Autodesk Inventor part; units mm, degrees
ref_plane "YZ Plane" through (0, 0, 0) normal (1, 0, 0) x (0, 1, 0)
ref_plane "XZ Plane" through (0, 0, 0) normal (0, 1, 0) x (-1, 0, 0)
ref_plane "XY Plane" through (0, 0, 0) normal (0, 0, 1) x (1, 0, 0)
sketch "Sketch1" plane through (0, 0, 0) normal (1, 0, 0) x (0, 1, 0)
  line L0 (0, 0) -> (3.5, 0)
  arc A0 (6.3262, -0.7277) -> (3.5, 0) centre (3.7831, -4.7528) ccw
  arc A1 (6.3262, -0.7277) -> (9.2314, -2.0228) centre (10.456, 4.6303) ccw
  line L1 (0, 0) -> (0, 0.25)
  line L2 (0, 0.25) -> (3.5, 0.25)
  line L3 (6.3262, -0.7277) -> (6.3262, -0.4777)
  line L4 (9.2314, -2.0228) -> (9.2314, -1.7728)
  arc A2 (6.3262, -0.4777) -> (3.5, 0.25) centre (3.658, -4.9886) ccw
  arc A3 (6.3262, -0.4777) -> (9.2314, -1.7728) centre (10.4213, 4.8026) ccw
  dimension "d0" = 3.5
  dimension "d1" = 0.25
  dimension "d2" = 3.5
  dimension "d3" = 0.25
  dimension "d4" = 0.25
extrude "Extrusion1" add sketch "Sketch1" along normal blind 5
properties part number "ribbonCable"
Verification items for the finished model (mm, model axes). Coordinates: 2 decimals unless noted, no trailing zeros. Order: outer loops, then holes, each group sorted by start corner. A loop starts at its lowest first (then second) coordinate and runs counter-clockwise, first axis right, second up. Notation, with made-up numbers: (69, 27.5) -> (128, 27.5) arc R7 cw to (128, 32.5) -> close; hole circle Ø5 at (7.25, 10.5). An arc over 180 degrees is marked (long way). Use CSV: the item, a comma, the result in double quotes. Start each with the question number.
Q1. Section check B-B, the plane z = 0.15. Record the cut outline in (x, y), and give its area (3 significant figures).
Q2. Depth check by flat-ended pin: P1, Ø3, axis at x = 1.5, y = 2, coming from the -Z side; P2, Ø3, axis at x = 1, y = 4.5, coming from the -Z side; P3, Ø1, axis at x = 2.5, y = 2, coming from the +Z side. Enter the tip coordinate at first touch or a pass-through.
Q3. Thickness scan on line 1 along Z through (x, y) = (2.1, 3.5); line 2 along Y through (x, z) = (2.75, -0.4). Record the ranges inside material, lowest first.
Q4. Section check A-A, the plane x = 0.3. Record the cut outline in (y, z), and give its area (3 significant figures).
Q5. Draft check along Y on faces 1 (the cylindrical face through (2.465, 7.722, -1.558)), 2 (the cylindrical face through (2.5, 7.7, -1.3)), 3 (the flat face through (2, 2, 0)). Enter one of: +Y half, -Y half, draft (parallel to the pull), parting line (faces both ways), or undercut.
Q6. Section check C-C, the plane y = 7.75. Record the cut outline in (x, z).
Returned:
1,outline,"(0, 0) -> (5, 0) -> (5, 4.69) -> (0, 4.69) -> close"
1,area,"23.4 mm^2"
2,P1,"stops at z = 0"
2,P2,"stops at z = -0.54"
2,P3,"stops at z = 0.25"
3,line 1,"z = 0 to 0.25"
3,line 2,"y = 5.71 to 6.19"
4,outline,"(0, 0) -> (3.5, 0) arc R4.76 cw to (6.33, -0.73) arc R6.76 ccw to (9.23, -2.02) -> (9.23, -1.77) arc R6.68 cw to (6.33, -0.48) arc R5.24 ccw to (3.5, 0.25) -> (0, 0.25) -> close"
4,area,"2.26 mm^2"
5,face 1,"-Y half"
5,face 2,"+Y half"
5,face 3,"draft"
6,outline,"(0, -1.57) -> (5, -1.57) -> (5, -1.32) -> (0, -1.32) -> close"
